Build history of the part. All positions in model axes, mm. A direction names the side the tool comes from. Coordinates: 2 decimals unless noted, no trailing zeros. Write each loop counter-clockwise with the first axis right and the second up, starting at its lowest first coordinate (ties: lowest second). Pieces come first, ordered by that corner, then holes.
```python
from build123d import *

# Parameters (mm, degrees)
F0_W     = 7.9
F0_H     = 2.45
F1_DEPTH = 0.5
F2_R     = 0.2
F3_W     = 4
F3_H     = 2.1
F4_DEPTH = 1
F5_R     = 0.2
F6_W     = 3.5
F6_H     = 1.6
F7_DEPTH = 0.1


with BuildPart() as f1:
    # F0 (on Top) → F1 (new body)
    with BuildSketch(Plane.XY):
        Rectangle(F0_W, F0_H)
    extrude(amount=F1_DEPTH)

    # F2
    f2_edges = [f1.edges().sort_by_distance(p)[0] for p in [
        (-3.95, -1.225, 0.25),
        (3.95, -1.225, 0.25),
        (3.95, 1.225, 0.25),
        (-3.95, 1.225, 0.25),
    ]]
    fillet(f2_edges, radius=F2_R)

    # F3 (on face) → F4 (join)
    with BuildSketch(Plane.XY.offset(0.5)):
        Rectangle(F3_W, F3_H)
    extrude(amount=F4_DEPTH)

    # F5
    f5_edges = [f1.edges().sort_by_distance(p)[0] for p in [
        (-2, -1.05, 1),
        (2, -1.05, 1),
        (2, 1.05, 1),
        (-2, 1.05, 1),
    ]]
    fillet(f5_edges, radius=F5_R)

    # F6 (on face) → F7 (join)
    with BuildSketch(Plane.XY.offset(1.5)):
        Rectangle(F6_W, F6_H)
    extrude(amount=F7_DEPTH)


solid = f1.part
```
1. Saw through at D-D on x = -2.25. List the corners of the cut face in (y, z) (3 decimals).
Computed values:
outline: (-1.225, 0) - (1.225, 0) - (1.225, 0.5) - (-1.225, 0.5) - close
2. Saw through at B-B on y = 0.7. List the corners of the cut face in (x, z).
Computed values:
outline: (-3.95, 0) - (3.95, 0) - (3.95, 0.5) - (2, 0.5) - (2, 1.5) - (1.75, 1.5) - (1.75, 1.6) - (-1.75, 1.6) - (-1.75, 1.5) - (-2, 1.5) - (-2, 0.5) - (-3.95, 0.5) - close
3. Saw through at A-A on x = -1.25. List the corners of the cut face in (y, z) (3 decimals), plus the area to 4 significant figures.
Computed values:
outline: (-1.225, 0) - (1.225, 0) - (1.225, 0.5) - (1.05, 0.5) - (1.05, 1.5) - (0.8, 1.5) - (0.8, 1.6) - (-0.8, 1.6) - (-0.8, 1.5) - (-1.05, 1.5) - (-1.05, 0.5) - (-1.225, 0.5) - close
area: 3.485 mm2
4. Probe line 1 along X through (y, z) = (-0.6, 0.8); line 2 along Z through (x, y) = (3, -0.65); line 3 along Y through (x, z) = (0.25, 1.05). List the from-to ranges inside material, lowest first.
Computed values:
line 1: x = -2 to 2
line 2: z = 0 to 0.5
line 3: y = -1.05 to 1.05
5. Saw through at C-C on z = 1.1. List the corners of the cut face in (x, y).
Computed values:
outline: (-2, -0.85) arc R0.2 ccw to (-1.8, -1.05) - (1.8, -1.05) arc R0.2 ccw to (2, -0.85) - (2, 0.85) arc R0.2 ccw to (1.8, 1.05) - (-1.8, 1.05) arc R0.2 ccw to (-2, 0.85) - close
6. Flat gauge pins, fed straight in: pin 1 (0.8 mm diameter, centred on y = 0, z = 1, fed in from +X); pin 2 (0.5 mm diameter, centred on x = 0, z = 1, fed in from -Y). Where does each tip first touch, or does it go through?
Computed values:
pin 1: stops at x = 2
pin 2: stops at y = -1.05
7. 3-axis set-ups, long thin cutter, end or side, ignore diameter. For faces 1 (the face through (0, -1.05, 1)), 2 (the face through (2, 0, 1)), 3 (the face through (0, 1.05, 1)): which of +Z, -Z, +X, -X, +Y, -Y reach the whole face in a straight line?
Computed values:
face 1: +Z, +X, -X, -Y
face 2: +Z, +X, +Y, -Y
face 3: +Z, +X, -X, +Y
